from build123d import *

# Parameters (mm, degrees)
F1_DEPTH = 43.18
F2_W     = 13.722286
F2_H     = 9.405698
F3_DEPTH = 25.4


with BuildPart() as f1:
    # F0 (on Front) → F1 (new body)
    with BuildSketch(Plane.XZ):
        Polygon((0, 49.633805), (0, 0), (76.640435, 0), (76.640435, 49.633805), (62.918149, 49.633805), (62.918149, 11.386576), (38.320217, 11.386576), (13.284341, 11.386576), (13.284341, 49.633805), align=None)
    extrude(amount=F1_DEPTH)

    # F2 (on face) → F3 (cut)
    with BuildSketch(Plane.XY.offset(49.633805)):
        with Locations((69.779292, -21.59)):
            Rectangle(F2_W, F2_H)
    extrude(amount=-F3_DEPTH, mode=Mode.SUBTRACT)


solid = f1.part
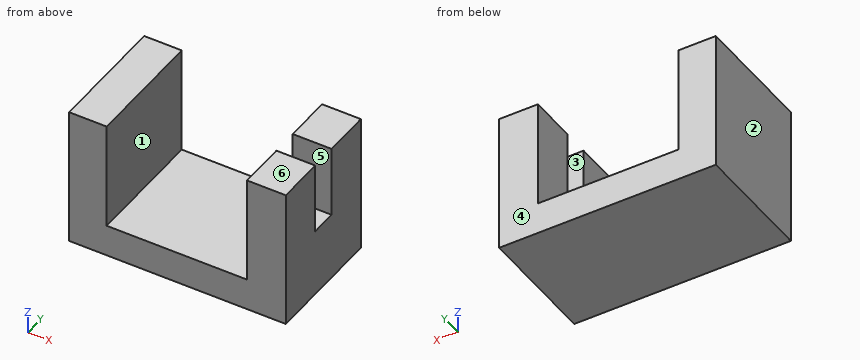
Design review of the part built by this model. Coordinates are the model's own, in mm. Face numbers are marked on the shaded views. A direction names the side the tool comes from. Give positions to 0.01 mm unless a question says otherwise; leave off trailing zeros. Order: outer loops, then holes, each group sorted by start corner. A loop starts at its lowest first (then second) coordinate and runs counter-clockwise, first axis right, second up.
1. Add section C-C, the plane y = -28.5. State the section outline as (x, z) points, then the cut area to 3 significant figures.
Solution:
outline: (0, 0) - (76.64, 0) - (76.64, 49.63) - (62.92, 49.63) - (62.92, 11.39) - (13.28, 11.39) - (13.28, 49.63) - (0, 49.63) - close
area: 1,910 mm2
2. Add section D-D, the plane x = 66. State the section outline as (y, z) points.
Solution:
outline: (-43.18, 0) - (0, 0) - (0, 49.63) - (-16.89, 49.63) - (-16.89, 24.23) - (-26.29, 24.23) - (-26.29, 49.63) - (-43.18, 49.63) - close
3. Add section A-A, the plane z = 42. State the section outline as (x, y) points.
Solution:
outline: (0, -43.18) - (13.28, -43.18) - (13.28, 0) - (0, 0) - close; (62.92, -43.18) - (76.64, -43.18) - (76.64, -26.29) - (62.92, -26.29) - close; (62.92, -16.89) - (76.64, -16.89) - (76.64, 0) - (62.92, 0) - close
4. Tool access review of the marked faces 1 and 2: name each direction out of +Z, -Z, +X, -X, +Y, -Y from which nothing blocks a thin tool from reaching the whole face with its end or side.
Solution:
face 1: +Z, +Y, -Y
face 2: +Z, -Z, -X, +Y, -Y
5. To check wall thickness, follow L1, parallel to X at y = -14, z = 14.5; L2, parallel to Z at x = 70.5, y = -20; L3, parallel to Z at x = 18.5, y = -19. State the ranges of each line that lie inside material, in increasing order.
Solution:
L1: x = 0 to 13.28, 62.92 to 76.64
L2: z = 0 to 24.23
L3: z = 0 to 11.39
6. Add section B-B, the plane z = 23. State the section outline as (x, y) points.
Solution:
outline: (0, -43.18) - (13.28, -43.18) - (13.28, 0) - (0, 0) - close; (62.92, -43.18) - (76.64, -43.18) - (76.64, 0) - (62.92, 0) - close
7. For pin 1 Ø19 at (y, z) = (-17.5, 29) entering from +X; pin 2 Ø3 at (x, y) = (71.5, -20.5) entering from +Z; pin 3 Ø13 at (x, y) = (32.5, -29.5) entering from +Z, all flat-tipped, find the tip position at first contact; note any pin that passes through.
Solution:
pin 1: stops at x = 76.64
pin 2: stops at z = 24.23
pin 3: stops at z = 11.39
8. Mouldability with a two-part tool opening along Y and no side actions: class the marked faces 3, 4, 5 and 6 as +Y half, -Y half, draft (parallel to the pull), parting line (faces both ways), or undercut.
Solution:
face 3: undercut
face 4: +Y half
face 5: undercut
face 6: draft
